Geometry: final body of the model. Coordinates: model frame, mm. A direction names the side the tool comes from. Round coordinates to 2 decimals unless told otherwise and drop trailing zeros. Order: outer loops, then holes, each group sorted by start corner. A loop starts at its lowest first (then second) coordinate and runs counter-clockwise, first axis right, second up. Notation, with made-up numbers: (-24, 51.5) -> (-10, 51.5) arc R26 ccw to (-10, 88.5) -> close; hole circle Ø5 at (-11, 12). An arc over 180 degrees is marked (long way). Put each result on its own line as item: value.
```python
from build123d import *

# Parameters (mm, degrees)
SKETCH1_R           = 2.5
BOSS_EXTRUDE1_DEPTH = 43.5
SKETCH2_R           = 5
BOSS_EXTRUDE2_DEPTH = 5
CUT_EXTRUDE2_START  = 10
SKETCH3_R           = 1.75
CUT_EXTRUDE2_DEPTH  = 20


with BuildPart() as part:
    # Sketch1 → Boss-Extrude1 (new body)
    with BuildSketch(Plane.XY):
        Circle(SKETCH1_R)
    extrude(amount=BOSS_EXTRUDE1_DEPTH)

    # Sketch2 → Boss-Extrude2 (add)
    with BuildSketch(Plane.XY.offset(43.5)):
        Circle(SKETCH2_R)
    extrude(amount=BOSS_EXTRUDE2_DEPTH)

    # Sketch3 → Cut-Extrude2 (cut)
    with BuildSketch(Plane(origin=(0, 0, 0), x_dir=(0, 0, -1), z_dir=(1, 0, 0)).offset(CUT_EXTRUDE2_START)):
        with Locations(Location((-10.5, 0, 0), (0, 0, 180))):
            Circle(SKETCH3_R)
    extrude(amount=-CUT_EXTRUDE2_DEPTH, mode=Mode.SUBTRACT)


solid = part.part
```
1. Material intervals for probe 1 along Z at (x, y) = (-1.5, 3.25); probe 2 along Y at (x, z) = (0.4, 10.5); probe 3 along Z at (x, y) = (0.75, -1.5), sorted ascending.
Ans:
probe 1: 43.5 to 48.5
probe 2: -2.47 to -1.75, 1.75 to 2.47
probe 3: 0 to 9.6, 11.4 to 48.5
2. Cut plane D-D on z = 45. Return loops of the section in (x, y).
Ans:
outline: circle Ø10 at (0, 0)
3. Contact query for flat-ended pins moving along their axis: P1, Ø6, axis at x = 1.5, z = 24, coming from the -Y side; P2, Ø5, axis at y = 3.5, z = 18, coming from the -X side; P3, Ø3, axis at y = 0, z = 10.5, coming from the -X side. Output: stop coordinate, or through.
Ans:
P1: y = -2.5
P2: x = -2.29
P3: through
4. Cut plane C-C on z = 10.5. Return loops of the section in (x, y).
Ans:
outline: (-1.79, -1.75) arc R2.5 ccw to (1.79, -1.75) -> close; (-1.79, 1.75) -> (1.79, 1.75) arc R2.5 ccw to start
5. Set-up query: faces 1 (the face through (-2.5, 0.1, 21.4)), 2 (the face through (0, 0, 0)). Return all of +Z, -Z, +X, -X, +Y, -Y with unobstructed straight access to the full face (end or side cutting, diameter ignored); none if empty.
Ans:
face 1: -Z
face 2: -Z, +X, -X, +Y, -Y
6. Cut plane B-B on y = 0.5. Return loops of the section in (x, z), and give its area (3 significant figures).
Ans:
outline: (-4.97, 43.5) -> (-2.45, 43.5) -> (-2.45, 12.18) -> (2.45, 12.18) -> (2.45, 43.5) -> (4.97, 43.5) -> (4.97, 48.5) -> (-4.97, 48.5) -> close; (-2.45, 0) -> (2.45, 0) -> (2.45, 8.82) -> (-2.45, 8.82) -> close
area: 246 mm²
7. Cut plane A-A on x = 0. Return loops of the section in (y, z), and give its area (3 significant figures).
Ans:
outline: (-5, 43.5) -> (-2.5, 43.5) -> (-2.5, 0) -> (2.5, 0) -> (2.5, 43.5) -> (5, 43.5) -> (5, 48.5) -> (-5, 48.5) -> close; hole circle Ø3.5 at (0, 10.5)
area: 258 mm²
